Here's how the part is built. I have some questions about the finished solid (model axes, mm). A direction names the side the tool comes from. Round coordinates to 2 decimals unless told otherwise and drop trailing zeros. Order: outer loops, then holes, each group sorted by start corner. A loop starts at its lowest first (then second) coordinate and runs counter-clockwise, first axis right, second up.
```python
from build123d import *

# Parameters (mm, degrees)
F0_W        = 2
F0_H        = 0.5
F1_DEPTH    = 11
F2_T1_DEPTH = 17.8819096024
F2_T3_DEPTH = 16
F2_T5_DEPTH = 14.63271264
F2_T7_DEPTH = 15.3301270189
F3_W        = 2
F3_H        = 3
F4_DEPTH    = 15


# Not quite as in the source:
# - a fillet or chamfer that OpenCascade refuses, or shapes differently, is made with other operations: its cross-section is extruded or revolved along the edge and cut away or added


with BuildPart() as f1:
    # F0 (on Top) → F1 (new body)
    with BuildSketch(Plane.XY):
        with BuildLine():
            Line((-14.1, 9.4475987206), (-14.1, 0))
            ThreePointArc((-14.1, 0), (0, -14.1), (14.1, 0))
            Line((14.1, 0), (14.1, 9.4475987206))
            Line((14.1, 9.4475987206), (12.1, 9.4475987206))
            Line((12.1, 9.4475987206), (10.2, 3.6))
            Line((10.2, 3.6), (12.6, 3.6))
            Line((12.6, 3.6), (12.6, 0))
            Line((12.6, 0), (9.5, 0))
            Line((9.5, 0), (7.5, 0))
            Line((7.5, 0), (0, 0))
            Line((0, 0), (-7.5, 0))
            Line((-7.5, 0), (-9.5, 0))
            Line((-9.5, 0), (-12.6, 0))
            Line((-12.6, 0), (-12.6, 3.6))
            Line((-12.6, 3.6), (-10.2, 3.6))
            Line((-10.2, 3.6), (-12.1, 9.4475987206))
            Line((-12.1, 9.4475987206), (-14.1, 9.4475987206))
        make_face()
        with BuildLine():
            ThreePointArc((12.4402572321, -2), (0, -12.6), (-12.4402572321, -2))
            Line((-12.4402572321, -2), (12.4402572321, -2))
        make_face(mode=Mode.SUBTRACT)
        with Locations((-8.5, 0.25)):
            Rectangle(F0_W, F0_H)
        with Locations((8.5, 0.25)):
            Rectangle(F0_W, F0_H)
    extrude(amount=F1_DEPTH)

    # F2: fillet of radius 1 on 10 edges, made by hand

    # F2_s2 → F2_t1 (cut)
    with BuildSketch(Plane.XY.offset(-3.4409548012)):
        with BuildLine():
            ThreePointArc((-11.5763819205, 3.6), (-10.7673649261, 4.0122147477), (-10.6253254042, 4.9090169944))
            Line((-10.6253254042, 4.9090169944), (-10.2, 3.6))
            Line((-10.2, 3.6), (-11.5763819205, 3.6))
        make_face()
        with BuildLine():
            ThreePointArc((10.6253254042, 4.9090169944), (10.7673649261, 4.0122147477), (11.5763819205, 3.6))
            Line((11.5763819205, 3.6), (10.2, 3.6))
            Line((10.2, 3.6), (10.6253254042, 4.9090169944))
        make_face()
    extrude(amount=F2_T1_DEPTH, mode=Mode.SUBTRACT)

    # F2_s4 → F2_t3 (cut)
    with BuildSketch(Plane.XY.offset(-2.5)):
        with BuildLine():
            ThreePointArc((-13.1, 9.4475987206), (-13.8071067812, 9.1547055018), (-14.1, 8.4475987206))
            Line((-14.1, 8.4475987206), (-14.1, 9.4475987206))
            Line((-14.1, 9.4475987206), (-13.1, 9.4475987206))
        make_face()
        with BuildLine():
            ThreePointArc((14.1, 8.4475987206), (13.8071067812, 9.1547055018), (13.1, 9.4475987206))
            Line((13.1, 9.4475987206), (14.1, 9.4475987206))
            Line((14.1, 9.4475987206), (14.1, 8.4475987206))
        make_face()
    extrude(amount=F2_T3_DEPTH, mode=Mode.SUBTRACT)

    # F2_s6 → F2_t5 (cut)
    with BuildSketch(Plane.XY.offset(-1.81635632)):
        with BuildLine():
            ThreePointArc((-11.8754860117, 8.756615715), (-12.2387572757, 9.256615715), (-12.826542528, 9.4475987206))
            Line((-12.826542528, 9.4475987206), (-12.1, 9.4475987206))
            Line((-12.1, 9.4475987206), (-11.8754860117, 8.756615715))
        make_face()
        with BuildLine():
            ThreePointArc((11.8754860117, 8.756615715), (12.2387572757, 9.256615715), (12.826542528, 9.4475987206))
            Line((12.826542528, 9.4475987206), (12.1, 9.4475987206))
            Line((12.1, 9.4475987206), (11.8754860117, 8.756615715))
        make_face()
    extrude(amount=F2_T5_DEPTH, mode=Mode.SUBTRACT)

    # F2_s8 → F2_t7 (cut)
    with BuildSketch(Plane.XY.offset(-2.1650635095)):
        with BuildLine():
            ThreePointArc((-8.6339745962, 0.5), (-9.1339745962, 0.3660254038), (-9.5, 0))
            Line((-9.5, 0), (-9.5, 0.5))
            Line((-9.5, 0.5), (-8.6339745962, 0.5))
        make_face()
        with BuildLine():
            ThreePointArc((-7.5, 0), (-7.8660254038, 0.3660254038), (-8.3660254038, 0.5))
            Line((-8.3660254038, 0.5), (-7.5, 0.5))
            Line((-7.5, 0.5), (-7.5, 0))
        make_face()
        with BuildLine():
            ThreePointArc((8.3660254038, 0.5), (7.8660254038, 0.3660254038), (7.5, 0))
            Line((7.5, 0), (7.5, 0.5))
            Line((7.5, 0.5), (8.3660254038, 0.5))
        make_face()
        with BuildLine():
            ThreePointArc((9.5, 0), (9.1339745962, 0.3660254038), (8.6339745962, 0.5))
            Line((8.6339745962, 0.5), (9.5, 0.5))
            Line((9.5, 0.5), (9.5, 0))
        make_face()
    extrude(amount=F2_T7_DEPTH, mode=Mode.SUBTRACT)

    # F3 (on Right) → F4 (cut, symmetric)
    with BuildSketch(Plane.YZ):
        with Locations((-3, 5.5)):
            Rectangle(F3_W, F3_H)
        with Locations((8.4475987206, 5.5)):
            Rectangle(F3_W, F3_H)
    extrude(amount=F4_DEPTH, both=True, mode=Mode.SUBTRACT)


solid = f1.part
```
1. If we section it at D-D, the plane z = 7.5: Write out the boundary of the cut face in (x, y), and give its area (3 significant figures).
Evaluation:
outline: (-14.1, 0) arc R14.1 ccw to (14.1, 0) - (14.1, 8.45) arc R1 ccw to (13.1, 9.45) - (12.83, 9.45) arc R1 ccw to (11.88, 8.76) - (10.63, 4.91) arc R1 ccw to (11.58, 3.6) - (12.6, 3.6) - (12.6, 0) - (9.5, 0) arc R1 ccw to (8.63, 0.5) - (8.37, 0.5) arc R1 ccw to (7.5, 0) - (-7.5, 0) arc R1 ccw to (-8.37, 0.5) - (-8.63, 0.5) arc R1 ccw to (-9.5, 0) - (-12.6, 0) - (-12.6, 3.6) - (-11.58, 3.6) arc R1 ccw to (-10.63, 4.91) - (-11.88, 8.76) arc R1 ccw to (-12.83, 9.45) - (-13.1, 9.45) arc R1 ccw to (-14.1, 8.45) - close; hole (-12.44, -2) arc R12.6 ccw to (12.44, -2) - close
area: 158 mm2
2. If we mould it in two halves opening along Y, with no side actions, what happens to faces 1 (the flat face through (-12, 3.6, 5)), 2 (the flat face through (-11.242, 6.806, 5.423)), 3 (the flat face through (-1, -1, 0))? For each: released by +Y, released by -Y, zero draft, split by the parting line, or undercut.
Evaluation:
face 1: undercut
face 2: released by +Y
face 3: zero draft
3. If we section it at A-A, the plane x = 0: Write out the boundary of the cut face in (y, z).
Evaluation:
outline: (-14.1, 0) - (-12.6, 0) - (-12.6, 11) - (-14.1, 11) - close; (-2, 0) - (0, 0) - (0, 11) - (-2, 11) - close
4. I need wall thicknesses on probe 1 along X at (y, z) = (1.5, 4.75); probe 2 along Y at (x, z) = (2, 7.5); probe 3 along Y at (x, z) = (-0.5, 3). Which ranges of each line are inside material? Lowest first, please.
Evaluation:
probe 1: x = -14.1 to -12.6, 12.6 to 14.1
probe 2: y = -13.96 to -12.44, -2 to 0
probe 3: y = -14.09 to -12.59, -2 to 0
5. If we section it at C-C, the plane y = -5.25: Write out the boundary of the cut face in (x, z).
Evaluation:
outline: (-13.09, 0) - (-11.45, 0) - (-11.45, 11) - (-13.09, 11) - close; (11.45, 0) - (13.09, 0) - (13.09, 11) - (11.45, 11) - close
6. I'm going to push flat-ended pins straight in: P1, Ø0.8, axis at x = -13, z = 5, coming from the +Y side; P2, Ø2, axis at y = -10, z = 4, coming from the -X side; P3, Ø8, axis at x = 5, y = 5.5, coming from the -Z side; P4, Ø1, axis at y = -2.5, z = 1.5, coming from the +X side. Where does each tip first touch, or does it pass through?
Evaluation:
P1: stops at y = 7.45
P2: stops at x = -10.85
P3: passes through
P4: stops at x = 13.96
7. If we section it at B-B, the plane z = 5.5: Write out the boundary of the cut face in (x, y), and give its area (3 significant figures).
Evaluation:
outline: (-14.1, 0) arc R14.1 ccw to (-13.96, -2) - (13.96, -2) arc R14.1 ccw to (14.1, 0) - (14.1, 7.45) - (11.45, 7.45) - (10.63, 4.91) arc R1 ccw to (11.58, 3.6) - (12.6, 3.6) - (12.6, 0) - (9.5, 0) arc R1 ccw to (8.63, 0.5) - (8.37, 0.5) arc R1 ccw to (7.5, 0) - (-7.5, 0) arc R1 ccw to (-8.37, 0.5) - (-8.63, 0.5) arc R1 ccw to (-9.5, 0) - (-12.6, 0) - (-12.6, 3.6) - (-11.58, 3.6) arc R1 ccw to (-10.63, 4.91) - (-11.45, 7.45) - (-14.1, 7.45) - close; (-13.52, -4) arc R14.1 ccw to (13.52, -4) - (11.95, -4) arc R12.6 cw to (-11.95, -4) - close
area: 144 mm2
8. On a 3-axis mill with a long thin cutter (end or side, diameter ignored), from which of +Z, -Z, +X, -X, +Y, -Y can I reach the whole of each face in a straight line? I mean faces 4 (the flat face through (12, 3.6, 5)), 5 (the flat face through (13, 8, 4)), 6 (the flat face through (0, 0, 5)), 7 (the cylindrical face through (-13.8, 9.16, 8.97)), 8 (the flat face through (13, -3, 4)). Say none if no direction works.
Evaluation:
face 4: +Z, -Z
face 5: +X, -X, +Y
face 6: +Z, -Z, +Y
face 7: +Z, -Z, -X, +Y
face 8: +X, -X
